Autodesk Inventor part; units mm, degrees
ref_plane "YZ Plane" through (0, 0, 0) normal (1, 0, 0) x (0, 1, 0)
ref_plane "XZ Plane" through (0, 0, 0) normal (0, 1, 0) x (-1, 0, 0)
ref_plane "XY Plane" through (0, 0, 0) normal (0, 0, 1) x (1, 0, 0)
sketch "Esboço1" plane through (0, 0, 0) normal (0, 0, 1) x (1, 0, 0)
  line L0 (-10.1444, 2.75) -> (10.1444, 2.75)
  line L1 (-10.1444, -2.75) -> (10.1444, -2.75)
  circle A0 centre (-14.9075, 0) radius 5.5
  circle A1 centre (14.9075, 0) radius 5.5
  circle A2 centre (-14.9075, 0) radius 3.5
  circle A3 centre (14.9075, 0) radius 3.5
  point P0 (0, 0)
  point P1 (0, 2.75)
  point P2 (0, -2.75)
  dimension "d7" = 11
  dimension "d5" = 2.75
  dimension "d6" = 2.75
  dimension "d9" = 14.9075
  dimension "d11" = 29.815
  dimension "d12" = 7
  dimension "d13" = 7
extrude "Extrusão1" add sketch "Esboço1" along normal mid plane 3.9 contours L0 A1 L1 A0 | A0 | A1 | A2 | A3
sketch "Esboço2" plane through (0, 0, -1.95) normal (0, 0, -1) x (-1, 0, 0)
  line L0 (-7.7154, -2.75) -> (7.7154, -2.75)
  line L1 (7.7154, -2.75) -> (7.7154, 2.75)
  line L2 (7.7154, 2.75) -> (-7.7154, 2.75)
  line L3 (-7.7154, 2.75) -> (-7.7154, -2.75)
  line L4 (-7.7154, -2.75) -> (7.7154, 2.75) construction
  line L5 (7.7154, -2.75) -> (-7.7154, 2.75) construction
  line L6 (10.1444, 2.75) -> (-10.1444, 2.75)
  line L7 (-10.1444, -2.75) -> (10.1444, -2.75)
  point P0 (0, 0)
  point P1 (0, 2.75)
  point P2 (0, -2.75)
  point P3 (7.7154, 0)
  point P4 (0, 2.75)
  dimension "d21" = 15.4307
extrude "Extrusão2" add sketch "Esboço2" along normal blind 8.04
sketch "Esboço3" plane through (0, 0, 1.95) normal (0, 0, 1) x (1, 0, 0)
  arc A0 (10.1444, -2.75) -> (10.1444, 2.75) centre (14.9075, 0) ccw
  point P0 (0, 0)
hole "Furo1" at (14.9075, 0, 1.95) direction (0, 0, -1) diameter 3.5 end through all countersink diameter 7 countersink angle 82
sketch "Esboço4" plane through (0, 0, 1.95) normal (0, 0, 1) x (1, 0, 0)
  arc A0 (-10.1444, 2.75) -> (-10.1444, -2.75) centre (-14.9075, 0) ccw
  point P0 (0, 0)
hole "Furo2" at (-14.9075, 0, 1.95) direction (0, 0, -1) diameter 3.5 end through all countersink diameter 7 countersink angle 82
sketch "Esboço5" plane through (0, 0, -9.99) normal (0, 0, -1) x (-1, 0, 0)
  arc A0 (-10.1444, 2.75) -> (-10.1444, -2.75) centre (-14.9075, 0) ccw
  circle A1 centre (-14.9075, 0) radius 5.5
  arc A2 (10.1444, -2.75) -> (10.1444, 2.75) centre (14.9075, 0) ccw
  circle A3 centre (14.9075, 0) radius 5.5
  line L0 (-10.1444, 2.75) -> (10.1444, 2.75)
  line L1 (-10.1444, -2.75) -> (10.1444, -2.75)
  line L2 (-13.4641, 2.5) -> (-12.0207, 0)
  line L3 (-12.0207, 0) -> (-13.4641, -2.5)
  line L4 (-13.4641, -2.5) -> (-16.3509, -2.5)
  line L5 (-16.3509, -2.5) -> (-17.7943, 0)
  line L6 (-17.7943, 0) -> (-16.3509, 2.5)
  line L7 (-16.3509, 2.5) -> (-13.4641, 2.5)
  line L8 (16.3509, 2.5) -> (17.7943, 0)
  line L9 (17.7943, 0) -> (16.3509, -2.5)
  line L10 (16.3509, -2.5) -> (13.4641, -2.5)
  line L11 (13.4641, -2.5) -> (12.0207, 0)
  line L12 (12.0207, 0) -> (13.4641, 2.5)
  line L13 (13.4641, 2.5) -> (16.3509, 2.5)
  point P0 (0, 0)
  point P1 (-14.9075, 2.5)
  point P2 (14.9075, 2.5)
  dimension "d37" = 11
  dimension "d38" = 3
  dimension "d39" = 3
extrude "Extrusão3" add sketch "Esboço5" along normal blind 3.9
properties part number "Barra1_0001_001" material "Titânio"
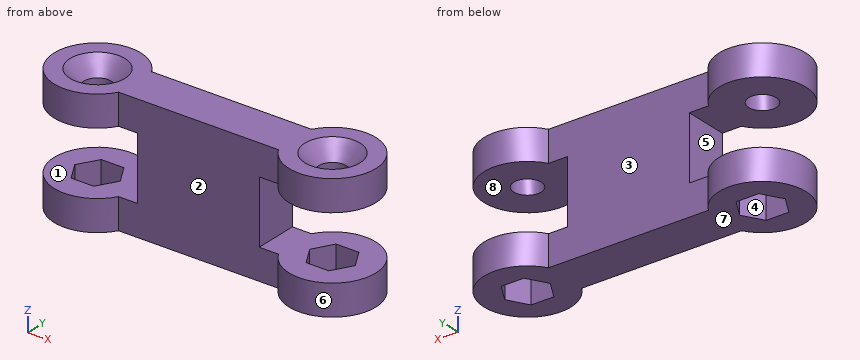
CAD build for the part. Positions are in the model's coordinates, mm. Face numbers are marked on the shaded views. A direction names the side the tool comes from. Give positions to 0.01 mm unless a question says otherwise; leave off trailing zeros. Loops run counter-clockwise (first coordinate to the right, second up) from the corner with the lowest first, then second, coordinate; pieces in that order, holes last. Notation, with made-up numbers: (81, 61) - (86, 61) arc R5 cw to (86, 67) - close; hole circle Ø11 at (65, 3.5). An arc over 180 degrees is marked (long way). Put each result on its own line as item: value.
Q1. Slice it at A-A (y = 5). Give the cut face in (x, z).
Filled in:
outline: (-17.2, -13.89) - (-12.62, -13.89) - (-12.62, -9.99) - (-17.2, -9.99) - close; (-17.2, -1.95) - (-12.62, -1.95) - (-12.62, 1.95) - (-17.2, 1.95) - close; (12.62, -13.89) - (17.2, -13.89) - (17.2, -9.99) - (12.62, -9.99) - close; (12.62, -1.95) - (17.2, -1.95) - (17.2, 1.95) - (12.62, 1.95) - close
Q2. Flat gauge pins, fed straight in: pin 1 (1 mm diameter, centred on x = -6, z = -3.5, fed in from +Y); pin 2 (3 mm diameter, centred on y = -0.5, z = -5, fed in from -X); pin 3 (2 mm diameter, centred on x = 14.91, y = 0, fed in from -Z). Where does each tip first touch, or does it go through?
Filled in:
pin 1: stops at y = 2.75
pin 2: stops at x = -7.72
pin 3: passes through
Q3. Slice it at C-C (x = -3). Give the cut face in (y, z), plus the area to 3 significant figures.
Filled in:
outline: (-2.75, -13.89) - (2.75, -13.89) - (2.75, 1.95) - (-2.75, 1.95) - close
area: 87.1 mm²
Q4. Slice it at B-B (z = -9.25). Give the cut face in (x, y), plus the area to 3 significant figures.
Filled in:
outline: (-7.72, -2.75) - (7.72, -2.75) - (7.72, 2.75) - (-7.72, 2.75) - close
area: 84.9 mm²
Q5. Slice it at D-D (y = -0.5). Give the number of separate pieces and of enclosed holes in the cut face, plus the area to 3 significant figures.
Filled in:
separate pieces: 5
enclosed holes: 0
area: 368 mm²
Q6. Probe line 1 along X through (y, z) = (0, -0.25); line 2 along Z through (x, y) = (-13, -3.75); line 3 along X through (y, z) = (0.5, -13). List the from-to ranges inside material, lowest first.
Filled in:
line 1: x = -20.41 to -16.66, -13.16 to 13.16, 16.66 to 20.41
line 2: z = -13.89 to -9.99, -1.95 to 1.95
line 3: x = -20.38 to -17.51, -12.31 to 12.31, 17.51 to 20.38
Q7. Tool access for the marked faces 1, 2, 3 and 4: list every direction of +Z, -Z, +X, -X, +Y, -Y with a clear straight run to the whole face (end or side of a thin tool).
Filled in:
face 1: -X, +Y, -Y
face 2: +Z, -Z, -Y
face 3: +Z, -Z, +Y
face 4: -Z
Q8. Mould opens along Z. For the marked faces 5, 6, 7 and 8 say: pulls with the +Z half, pulls with the -Z half, needs draft (parallel to the pull), parting line crosses it, or undercut.
Filled in:
face 5: undercut
face 6: needs draft
face 7: pulls with the -Z half
face 8: undercut
